Work out the finished part from the listing and answer in its coordinate system (mm). Face numbers are marked on the shaded views. Coordinates: 2 decimals unless noted, no trailing zeros. Write each question's results on one line, items separated by ' | '. Start each with the question number.
1. Find the intervals of material crossed by line 1 along Y through (x, z) = (27, -2.5); line 2 along X through (y, z) = (7, 44); line 3 along Y through (x, z) = (-14.5, 30.5), in increasing order. Write a range as [from, to].
2. Each of these flat-tipped pins is pushed along its axis until it touches: P1, Ø3, axis at y = -4.5, z = 33.5, coming from the -X side; P2, Ø10, axis at x = -30.5, z = 9.5, coming from the +Y side; P3, Ø4, axis at y = 25, z = 76.5, coming from the +X side. Where does it stop, or does it pass through?
3. Determine the mould class of the marked faces 1 and 2 for opening direction X: released by +X, released by -X, zero draft, split by the parting line, or undercut.
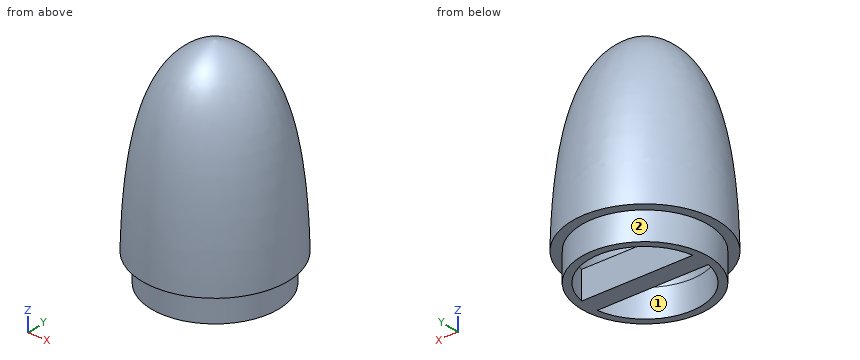
Autodesk Fusion 360 part; units mm, degrees
sketch "Sketch1" plane through (0, 0, 0) normal (1, 0, 0) x (0, 1, 0)
  line L0 (0, 0) -> (-39, 0) construction
  line L1 (0, 0) -> (0, 100) construction
  spline S0 degree 5 poles (-39, 0) (-38.942, 3.3768) (-38.7689, 10.0218) (-38.3385, 19.6635) (-37.4173, 31.8566) (-35.642, 45.9083) (-33.1709, 58.6335) (-29.9149, 69.8616) (-25.7862, 79.4253) (-20.7237, 87.2084) (-14.7404, 93.2356) (-9.2559, 96.7263) (-4.7703, 98.6346) (-1.6172, 99.5966) (0, 100) knots 0 0 0 0 0 0 0.1 0.2 0.3 0.4 0.5 0.6 0.7 0.8 0.9 1 1 1 1 1 1
  spline S1 degree 5 poles (-30, 0) (-30.0249, 3.0944) (-30.0256, 9.1895) (-29.8796, 18.0509) (-29.3857, 29.2944) (-28.2311, 42.3217) (-26.4766, 54.2023) (-24.0438, 64.7865) (-20.8549, 73.9254) (-16.8534, 81.5112) (-12.0463, 87.557) (-7.5889, 91.2244) (-3.9193, 93.3509) (-1.3302, 94.4957) (0, 95) knots 0 0 0 0 0 0 0.1 0.2 0.3 0.4 0.5 0.6 0.7 0.8 0.9 1 1 1 1 1 1
  line L2 (0, 95) -> (0, 100)
  line L3 (-30, 0) -> (-39, 0)
  point P0 (-25, 80)
  point P1 (-20, 75)
  dimension "d5" = 39
  dimension "d6" = 100
revolve "Revolve1" add sketch "Sketch1" angle 360 about axis through (0, 0, 0) along (0, 0, 1)
sketch "Sketch2" plane through (0, 0, 0) normal (0, 0, 1) x (1, 0, 0)
  circle A0 centre (0, 0) radius 34
  circle A1 centre (0, 0) radius 30
  dimension "d8" = 68
  dimension "d9" = 60
extrude "Extrude1" add sketch "Sketch2" against normal blind 15
sketch "Sketch3" plane through (0, 0, 0) normal (0, 0, 1) x (1, 0, 0)
  line L0 (-30, -5) -> (30, -5)
  line L1 (30, -5) -> (30, 5)
  line L2 (30, 5) -> (-30, 5)
  line L3 (-30, 5) -> (-30, -5)
extrude "Extrude2" add sketch "Sketch3" against normal blind 15
equation "innerdi = 68 mm"
equation "noseconeheight = 100 mm"
equation "d6 = noseconeheight"
equation "d8 = innerdi"
equation "d9 = innerdi - 8 mm"
Values:
1) line 1: [-20.66, -13.08], [-5, 5], [13.08, 20.66] | line 2: [-35.02, -26.95], [26.95, 35.02] | line 3: [-34.44, -25.29], [25.29, 34.44]
2) P1: x = -37.01 | P2: y = 29.17 | P3: x = 14.21
3) face 1: undercut | face 2: split by the parting line
